The model under review builds one solid part; all positions refer to its coordinate system, in mm. A direction names the side the tool comes from. Coordinates: 2 decimals unless noted, no trailing zeros. Order: outer loops, then holes, each group sorted by start corner. A loop starts at its lowest first (then second) coordinate and runs counter-clockwise, first axis right, second up.
```python
from build123d import *

# Parameters (mm, degrees)
F1_DEPTH  = 108
F3_DEPTH  = 150
F5_DEPTH  = 98
F7_DEPTH  = 100
F8_DEPTH  = 100
F10_DEPTH = 100
F11_R     = 10
F12_DEPTH = 25
F14_DEPTH = 100


with BuildPart() as f1:
    # F0 (on Top) → F1 (new body)
    with BuildSketch(Plane.XY):
        with BuildLine():
            Line((17.5, -50), (30, -50))
            Line((30, -50), (30, 47))
            ThreePointArc((30, 47), (29.1213203436, 49.1213203436), (27, 50))
            Line((27, 50), (-27, 50))
            ThreePointArc((-27, 50), (-29.1213203436, 49.1213203436), (-30, 47))
            Line((-30, 47), (-30, -50))
            Line((-30, -50), (-17.5, -50))
            Line((-17.5, -50), (-17.5, -48))
            Line((-17.5, -48), (-17.5, 48))
            Line((-17.5, 48), (17.5, 48))
            Line((17.5, 48), (17.5, -48))
            Line((17.5, -48), (17.5, -50))
        make_face()
    extrude(amount=F1_DEPTH)

    # F2 (on face) → F3 (cut)
    with BuildSketch(Plane.XZ.offset(50)):
        with BuildLine():
            Line((30, 0), (30, 25))
            ThreePointArc((30, 25), (26.4338203685, 10.8136283454), (16.5831239518, 0))
            Line((16.5831239518, 0), (30, 0))
        make_face()
        with BuildLine():
            ThreePointArc((-17.5, 0.633014138), (-26.6926956301, 11.3069360624), (-30, 25))
            Line((-30, 25), (-30, 0))
            Line((-30, 0), (-17.5, 0))
            Line((-17.5, 0), (-17.5, 0.633014138))
        make_face()
        with BuildLine():
            ThreePointArc((-16.5831239518, 0), (-17.0445009109, 0.3122502302), (-17.5, 0.633014138))
            Line((-17.5, 0.633014138), (-17.5, 0))
            Line((-17.5, 0), (-16.5831239518, 0))
        make_face()
    extrude(amount=-F3_DEPTH, mode=Mode.SUBTRACT)

    # F4 (on face) → F5 (cut)
    with BuildSketch(Plane.XZ.offset(50)):
        with BuildLine():
            ThreePointArc((-19.5, 45.0935312974), (-27.9682339411, 23.6666245026), (-17.5, 3.1425070056))
            Line((-17.5, 3.1425070056), (-17.5, 46.8574929944))
            ThreePointArc((-17.5, 46.8574929944), (-18.5210121272, 45.9993359367), (-19.5, 45.0935312974))
        make_face()
        with BuildLine():
            Line((17.5, 46.8574929944), (17.5, 3.1425070056))
            ThreePointArc((17.5, 3.1425070056), (25.2388589282, 12.875644347), (28, 25))
            ThreePointArc((28, 25), (25.7875939165, 35.9087121146), (19.5, 45.0935312974))
            ThreePointArc((19.5, 45.0935312974), (18.5210121272, 45.9993359367), (17.5, 46.8574929944))
        make_face()
    extrude(amount=-F5_DEPTH, mode=Mode.SUBTRACT)

    # F6 (on face) → F7 (cut)
    with BuildSketch(Plane.YZ.offset(30)):
        with BuildLine():
            Line((-50, 42.3148013651), (-50, 0))
            Line((-50, 0), (10, 0))
            ThreePointArc((10, 0), (-24.0239311691, 15.4516934038), (-50, 42.3148013651))
        make_face()
    extrude(amount=-F7_DEPTH, mode=Mode.SUBTRACT)

    # F4 (on face) → F8 (cut)
    with BuildSketch(Plane.XZ.offset(50)):
        with BuildLine():
            Line((-30, 108), (-30, 25))
            ThreePointArc((-30, 25), (-27.2488531869, 37.549900398), (-19.5, 47.7980262304))
            Line((-19.5, 47.7980262304), (-19.5, 108))
            Line((-19.5, 108), (-30, 108))
        make_face()
        with BuildLine():
            ThreePointArc((19.5, 47.7980262304), (27.2488531869, 37.549900398), (30, 25))
            Line((30, 25), (30, 108))
            Line((30, 108), (19.5, 108))
            Line((19.5, 108), (19.5, 47.7980262304))
        make_face()
    extrude(amount=-F8_DEPTH, mode=Mode.SUBTRACT)

    # F9 (on face) → F10 (cut)
    with BuildSketch(Plane.YZ.offset(19.5)):
        with BuildLine():
            ThreePointArc((-50, 62.7980262304), (-47.0710678119, 69.8690940422), (-40, 72.7980262304))
            Line((-40, 72.7980262304), (17.2408529371, 72.7980262304))
            ThreePointArc((17.2408529371, 72.7980262304), (24.311920749, 75.7269584185), (27.2408529371, 82.7980262304))
            Line((27.2408529371, 82.7980262304), (27.2408529371, 103))
            ThreePointArc((27.2408529371, 103), (28.7053190312, 106.5355339059), (32.2408529371, 108))
            Line((32.2408529371, 108), (-50, 108))
            Line((-50, 108), (-50, 62.7980262304))
        make_face()
    extrude(amount=-F10_DEPTH, mode=Mode.SUBTRACT)

    # F11 (on face) → F12 (cut)
    with BuildSketch(Plane(origin=(0, 50, 0), x_dir=(-1, 0, 0), z_dir=(0, 1, 0))):
        with Locations((0, 25)):
            Circle(F11_R)
    extrude(amount=-F12_DEPTH, mode=Mode.SUBTRACT)

    # F13 (on face) → F14 (cut)
    with BuildSketch(Plane(origin=(-19.5, 0, 0), x_dir=(0, -1, 0), z_dir=(-1, 0, 0))):
        with BuildLine():
            Line((35, 57.7980262304), (39.5, 57.7980262304))
            ThreePointArc((39.5, 57.7980262304), (38.1819805153, 60.9800067457), (35, 62.2980262304))
            Line((35, 62.2980262304), (35, 57.7980262304))
        make_face()
        with BuildLine():
            ThreePointArc((35, 62.2980262304), (31.8180194847, 54.616045715), (39.5, 57.7980262304))
            Line((39.5, 57.7980262304), (35, 57.7980262304))
            Line((35, 57.7980262304), (35, 62.2980262304))
        make_face()
    extrude(amount=-F14_DEPTH, mode=Mode.SUBTRACT)


solid = f1.part
```
(1) We need section B-B, the plane x = 0. Write out the cut boundary in (y, z), and give its area (3 significant figures).
A:
outline: (48, 0) - (50, 0) - (50, 15) - (48, 15) - close; (48, 35) - (50, 35) - (50, 108) - (48, 108) - close
area: 176 mm2
(2) Wall thickness on probe 1 along Z at (x, y) = (0, 49.2); probe 2 along X at (y, z) = (-26.5, 58.5); probe 3 along Y at (x, z) = (-16, 13): over which ranges is each line inside the solid? List them lowest first.
A:
probe 1: z = 0 to 15, 35 to 108
probe 2: x = -19.5 to -17.5, 17.5 to 19.5
probe 3: y = 48 to 50
(3) For pin 1 Ø1 at (x, y) = (18, -23) entering from +Z; pin 2 Ø10 at (y, z) = (-6, 49.5) entering from -X; pin 3 Ø0.6 at (x, z) = (-18, 95.5) entering from -Y; pin 4 Ø18 at (x, z) = (0, 25) entering from -Y, all flat-tipped, find the tip position at first contact; note any pin that passes through.
A:
pin 1: stops at z = 72.8
pin 2: stops at x = -22.8
pin 3: stops at y = 27.24
pin 4: passes through
(4) We need section D-D, the plane z = 86. Write out the cut boundary in (x, y), and give its area (3 significant figures).
A:
outline: (-19.5, 27.24) - (-17.5, 27.24) - (-17.5, 48) - (17.5, 48) - (17.5, 27.24) - (19.5, 27.24) - (19.5, 50) - (-19.5, 50) - close
area: 161 mm2
(5) Draft analysis for pull direction X (two halves, no side actions). For faces 4 (the face through (-19.5, 10, 71)), 5 (the face through (28.748, 49.438, 24.817)), 6 (the face through (18.514, 24.234, 75.65)), 7 (the face through (17.5, 11, 70)), state which applies: released by +X, released by -X, zero draft, split by the parting line, or undercut.
A:
face 4: released by -X
face 5: released by +X
face 6: zero draft
face 7: undercut
(6) We need section C-C, the plane z = 32. Write out the cut boundary in (x, y), and give its area (3 significant figures).
A:
outline: (-29.17, -42.24) - (-27.11, -42.24) - (-27.11, 48) - (-7.14, 48) - (-7.14, 50) - (-27, 50) arc R3 ccw to (-29.17, 49.07) - close; (7.14, 48) - (27.11, 48) - (27.11, -42.24) - (29.17, -42.24) - (29.17, 49.07) arc R3 ccw to (27, 50) - (7.14, 50) - close
area: 459 mm2
(7) We need section A-A, the plane y = 37. Write out the cut boundary in (x, z).
A:
outline: (-19.5, 47.8) arc R30 ccw to (-17.5, 0.63) - (-17.5, 3.14) arc R28 cw to (-17.5, 46.86) - (-17.5, 108) - (-19.5, 108) - close; (17.5, 0.63) arc R30 ccw to (19.5, 47.8) - (19.5, 108) - (17.5, 108) - (17.5, 46.86) arc R28 cw to (17.5, 3.14) - close
(8) Machinability: for faces 1 (the face through (-28.69, 49.48, 24.82)), 2 (the face through (0, 48, 53)), 3 (the face through (17.5, 24, 2)), which of the approach directions +Z, -Z, +X, -X, +Y, -Y give a long, thin tool a straight path to every point of the face, cutting with its end or side? Answer none if there is none.
A:
face 1: +Z, -Z, -X, +Y
face 2: -Y
face 3: +Z, -Z, -Y
